from build123d import *

# Parameters (mm, degrees)
F0_W     = 515
F0_H     = 120
F1_DEPTH = 90
F2_R     = 40
F3_DEPTH = 110
F4_R     = 12.5
F5_DEPTH = 25
F6_R     = 5
F7_DEPTH = 120
F8_DEPTH = 120


# Not quite as in the source:
# - a feature names something its author has since deleted; it is built from what else it names


with BuildPart() as f1:
    # F0 (on Right) → F1 (new body)
    with BuildSketch(Plane.YZ):
        Rectangle(F0_W, F0_H)
    extrude(amount=F1_DEPTH)

    # F2 (on face) → F3 (cut)
    with BuildSketch(Plane.XY.offset(60)):
        with Locations((45, 212.5)):
            Circle(F2_R)
        with Locations((45, 127.5)):
            Circle(F2_R)
        with Locations((45, 42.5)):
            Circle(F2_R)
        with Locations((45, -42.5)):
            Circle(F2_R)
        with Locations((45, -127.5)):
            Circle(F2_R)
        with Locations((45, -212.5)):
            Circle(F2_R)
    extrude(amount=-F3_DEPTH, mode=Mode.SUBTRACT)

    # F4 (on face) → F5 (cut)
    with BuildSketch(Plane.YZ.offset(90)):
        with Locations((-127.5, 32.5)):
            Circle(F4_R)
        with Locations((-212.5, 32.5)):
            Circle(F4_R)
        with Locations((-42.5, 32.5)):
            Circle(F4_R)
        with Locations((42.5, 32.5)):
            Circle(F4_R)
        with Locations((127.5, 32.5)):
            Circle(F4_R)
        with Locations((212.5, 32.5)):
            Circle(F4_R)
    extrude(amount=-F5_DEPTH, mode=Mode.SUBTRACT)

    # F6 (on face) → F7 (cut)
    with BuildSketch(Plane.XY.offset(60)):
        with Locations((80, 170)):
            Circle(F6_R)
        with Locations((80, 247.5)):
            Circle(F6_R)
        with Locations((80, 85)):
            Circle(F6_R)
        with Locations((10, 85)):
            Circle(F6_R)
        with Locations((10, 170)):
            Circle(F6_R)
        with Locations((10, 247.5)):
            Circle(F6_R)
        with Locations((80, 0)):
            Circle(F6_R)
        with Locations((80, -85)):
            Circle(F6_R)
        with Locations((10, -85)):
            Circle(F6_R)
        with Locations((10, -170)):
            Circle(F6_R)
        with Locations((80, -170)):
            Circle(F6_R)
        with Locations((80, -247.5)):
            Circle(F6_R)
        with Locations((10, -247.5)):
            Circle(F6_R)
    extrude(amount=-F7_DEPTH, mode=Mode.SUBTRACT)

    # F6 (on face) → F8 (cut)
    with BuildSketch(Plane.XY.offset(60)):
        with Locations((10, 0)):
            Circle(F6_R)
    extrude(amount=-F8_DEPTH, mode=Mode.SUBTRACT)


solid = f1.part
The model under review builds one solid part; all positions refer to its coordinate system, in mm. A direction names the side the tool comes from. Coordinates: 2 decimals unless noted, no trailing zeros. Loops run counter-clockwise (first coordinate to the right, second up) from the corner with the lowest first, then second, coordinate; pieces in that order, holes last.
(1) Insertion check: P1, Ø20, axis at y = -42.5, z = 32.5, coming from the +X side; P2, Ø5, axis at x = 58, y = 67.5, coming from the +Z side. Each pin has a flat end and moves straight along its axis. Give the tip position at first contact, or say it passes through.
Determined:
P1: stops at x = 6.27
P2: stops at z = -50
(2) Consider section B-B, the plane z = -29. Give the number of separate pieces and of enclosed holes in the cut face, plus the area to 3 significant figures.
Determined:
separate pieces: 1
enclosed holes: 20
area: 15,100 mm2
(3) Tool access review of faces 1 (the cylindrical face through (87.326, -115.953, 27.712)), 2 (the cylindrical face through (13.26, -151.84, 5.77)), 3 (the cylindrical face through (14.77, 1.5, 0.84)): name each direction out of +Z, -Z, +X, -X, +Y, -Y from which nothing blocks a thin tool from reaching the whole face with its end or side.
Determined:
face 1: +X
face 2: +Z
face 3: +Z, -Z
(4) Consider section A-A, the plane y = -212.5. Give the boundary of the cut face in (x, z), plus the area to 4 significant figures.
Determined:
outline: (0, -60) - (90, -60) - (90, 20) - (85, 20) - (85, -50) - (5, -50) - (5, 60) - (0, 60) - close; (85, 45) - (90, 45) - (90, 60) - (85, 60) - close
area: 1,875 mm2
(5) Draft analysis for pull direction Z (two halves, no side actions). For faces 4 (the flat face through (44, -42, -50)), 5 (the cylindrical face through (87.326, -30.953, 27.712)), 6 (the cylindrical face through (84.619, 83.085, 0.84)), state which applies: +Z half, -Z half, draft (parallel to the pull), parting line (faces both ways), or undercut.
Determined:
face 4: +Z half
face 5: undercut
face 6: draft
(6) Wall thickness on L1, parallel to X at y = -44.5, z = -36; L2, parallel to Z at x = 51, y = 161.5; L3, parallel to X at y = -135, z = -2.5: over which ranges is each line inside the solid? List them lowest first.
Determined:
L1: x = 0 to 5.05, 84.95 to 90
L2: z = -60 to -50
L3: x = 0 to 5.71, 84.29 to 90
(7) Consider section D-D, the plane y = -154. Give the boundary of the cut face in (x, z), plus the area to 3 significant figures.
Determined:
outline: (0, -60) - (90, -60) - (90, 60) - (74.96, 60) - (74.96, -50) - (15.04, -50) - (15.04, 60) - (0, 60) - close
area: 4,210 mm2
(8) Consider section C-C, the plane x = 55. Give the boundary of the cut face in (y, z), plus the area to 3 significant figures.
Determined:
outline: (-257.5, -60) - (257.5, -60) - (257.5, 60) - (251.23, 60) - (251.23, -50) - (173.77, -50) - (173.77, 60) - (166.23, 60) - (166.23, -50) - (88.77, -50) - (88.77, 60) - (81.23, 60) - (81.23, -50) - (3.77, -50) - (3.77, 60) - (-3.77, 60) - (-3.77, -50) - (-81.23, -50) - (-81.23, 60) - (-88.77, 60) - (-88.77, -50) - (-166.23, -50) - (-166.23, 60) - (-173.77, 60) - (-173.77, -50) - (-251.23, -50) - (-251.23, 60) - (-257.5, 60) - close
area: 10,700 mm2
